Check sheet for the drawn part. Datum: minimum x, y, z corner. Units: mm. Coordinates: 2 decimals unless noted, no trailing zeros. Loops run counter-clockwise (first coordinate to the right, second up) from the corner with the lowest first, then second, coordinate; pieces in that order, holes last. Notation, with made-up numbers: (87.25, -29.75) - (126.25, -29.75) arc R21 ccw to (126.25, -20.75) - close; hole circle Ø8 at (74.25, -34.75). An arc over 180 degrees is marked (long way). Answer as a JSON object with one key per item and string values. Group by question number.
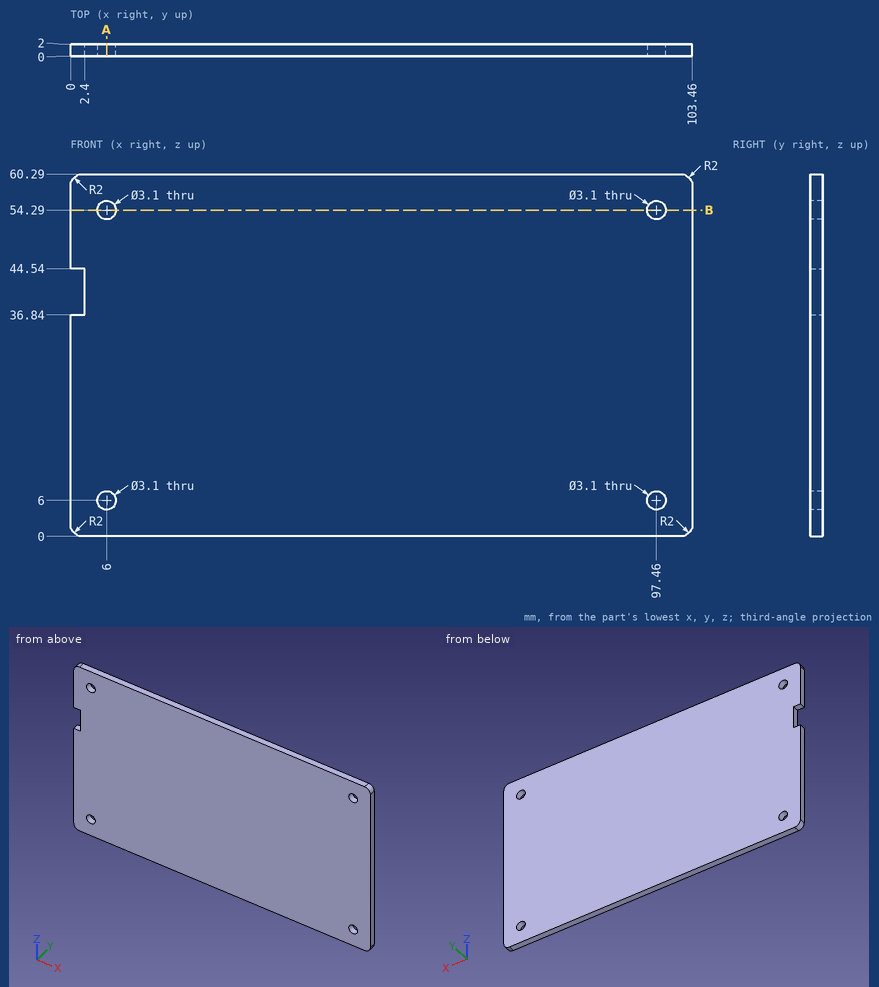
1. Sectioned sample at A-A on x = 6. Record the cut outline in (y, z).
2. Material ranges on line 1 (Z direction, x = 97.46, y = 0.5); line 2 (X direction, y = 0.65, z = 54.29); line 3 (Z direction, x = 96.5, y = 0.45), recorded low to high.
3. Sectioned sample at B-B on z = 54.29. Record the cut outline in (x, y), plus the area to 3 significant figures.
Answers follow:
{
 "1": {"outline": "(0, 0) - (2, 0) - (2, 4.45) - (0, 4.45) - close; (0, 7.55) - (2, 7.55) - (2, 52.74) - (0, 52.74) - close; (0, 55.84) - (2, 55.84) - (2, 60.29) - (0, 60.29) - close"},
 "2": {"line 1": "z = 0 to 4.45, 7.55 to 52.74, 55.84 to 60.29", "line 2": "x = 0 to 4.45, 7.55 to 95.91, 99.01 to 103.46", "line 3": "z = 0 to 4.78, 7.22 to 53.07, 55.51 to 60.29"},
 "3": {"outline": "(0, 0) - (4.45, 0) - (4.45, 2) - (0, 2) - close; (7.55, 0) - (95.91, 0) - (95.91, 2) - (7.55, 2) - close; (99.01, 0) - (103.46, 0) - (103.46, 2) - (99.01, 2) - close", "area": "195 mm^2"}
}
